```python
from build123d import *

# Parameters (mm, degrees)
MODEL_R             = 14.351
MODEL_R_2           = 2.413
MODEL_R_3           = 14.2875
BOSS_EXTRUDE1_DEPTH = 7.874
CUT_EXTRUDE3_REACH  = 9.874
SKETCH29_R          = 2.032
SKETCH29_R_2        = 9.525
CUT_EXTRUDE4_REACH  = 9.874
SKETCH34_R          = 2.4892
CUT_EXTRUDE5_REACH  = 9.874
SKETCH40_R          = 2.4892


with BuildPart() as part:
    # Model → Boss-Extrude1 (new body)
    with BuildSketch(Plane.XY):
        with BuildLine():
            Line((-44.522451968, 230.070582963), (-200.005250584, 313.419470721))
            ThreePointArc((-200.005250584, 313.419470721), (-219.438743814, 318.210854709), (-236.308771814, 307.439588539))
            Line((-236.308771814, 307.439588539), (-425.925316767, 28.829603592))
            ThreePointArc((-425.925316767, 28.829603592), (-430.312243104, 13.671313347), (-424.900993017, -1.152223962))
            Line((-424.900993017, -1.152223962), (-385.581467186, -51.204797614))
            ThreePointArc((-385.581467186, -51.204797614), (-376.711879358, -58.358090396), (-365.607528193, -60.913979882))
            Line((-365.607528193, -60.913979882), (-324.737451002, -60.913979882))
            ThreePointArc((-324.737451002, -60.913979882), (-318.798508014, -59.439796386), (-314.23831963, -55.359484793))
            Line((-314.23831963, -55.359484793), (-212.899365952, 93.541257838))
            ThreePointArc((-212.899365952, 93.541257838), (-203.778989185, 101.701881024), (-191.901103209, 104.650248016))
            Line((-191.901103209, 104.650248016), (48.661197018, 104.650248016))
            ThreePointArc((48.661197018, 104.650248016), (64.032332507, 99.471232012), (73.135172194, 86.046168785))
            Line((73.135172194, 86.046168785), (86.727013732, 37.098218434))
            ThreePointArc((86.727013732, 37.098218434), (106.362581421, 15.501750179), (127.326236921, 35.811553418))
            Line((127.326236921, 35.811553418), (140.807890588, 110.809453484))
            ThreePointArc((140.807890588, 110.809453484), (138.675228362, 126.361225539), (127.809114586, 137.689660276))
            Line((127.809114586, 137.689660276), (-44.522451968, 230.070582963))
        make_face()
        with Locations((-323.775189267, -35.513979882)):
            Circle(MODEL_R, mode=Mode.SUBTRACT)
        with Locations((-399.975189267, 2.586020118)):
            Circle(MODEL_R, mode=Mode.SUBTRACT)
        with Locations((107.006236921, 23.111553418)):
            Circle(MODEL_R_2, mode=Mode.SUBTRACT)
        with Locations((94.306236921, 35.811553418)):
            Circle(MODEL_R_2, mode=Mode.SUBTRACT)
        Polygon((110.67241113, 42.161553418), (114.33858534, 35.811553418), (110.67241113, 29.461553418), (103.340062712, 29.461553418), (99.673888502, 35.811553418), (103.340062712, 42.161553418), (107.006236921, 42.161553418), align=None, mode=Mode.SUBTRACT)
        with Locations((119.706236921, 35.811553418)):
            Circle(MODEL_R_2, mode=Mode.SUBTRACT)
        with Locations((107.006236921, 48.511553418)):
            Circle(MODEL_R_2, mode=Mode.SUBTRACT)
        with Locations((-190.707148919, 138.516914683)):
            Circle(MODEL_R, mode=Mode.SUBTRACT)
        with Locations((-208.832932893, 283.437784316)):
            Circle(MODEL_R, mode=Mode.SUBTRACT)
        with Locations((-40.935516122, 193.433854171)):
            Circle(MODEL_R_3, mode=Mode.SUBTRACT)
    extrude(amount=BOSS_EXTRUDE1_DEPTH)

    # Sketch29 → Cut-Extrude3 (cut, up to next)
    with BuildSketch(Plane.XY.offset(7.874), mode=Mode.PRIVATE) as cut_extrude3_sk1:
        with Locations((-182.711721066, 249.056735353)):
            Circle(SKETCH29_R)
    cut_extrude3_tool1 = extrude(cut_extrude3_sk1.sketch, amount=-CUT_EXTRUDE3_REACH, mode=Mode.PRIVATE) & part.part
    add(cut_extrude3_tool1.solids().sort_by_distance((-182.711721, 249.056735, 7.874))[0], mode=Mode.SUBTRACT)
    # Sketch29 → Cut-Extrude3 (cut, up to next)
    with BuildSketch(Plane.XY.offset(7.874), mode=Mode.PRIVATE) as cut_extrude3_sk2:
        with Locations((-134.081376724, 263.744472048)):
            Circle(SKETCH29_R)
    cut_extrude3_tool2 = extrude(cut_extrude3_sk2.sketch, amount=-CUT_EXTRUDE3_REACH, mode=Mode.PRIVATE) & part.part
    add(cut_extrude3_tool2.solids().sort_by_distance((-134.081377, 263.744472, 7.874))[0], mode=Mode.SUBTRACT)
    # Sketch29 → Cut-Extrude3 (cut, up to next)
    with BuildSketch(Plane.XY.offset(7.874), mode=Mode.PRIVATE) as cut_extrude3_sk3:
        with Locations((-165.740417242, 280.715775871)):
            Circle(SKETCH29_R)
    cut_extrude3_tool3 = extrude(cut_extrude3_sk3.sketch, amount=-CUT_EXTRUDE3_REACH, mode=Mode.PRIVATE) & part.part
    add(cut_extrude3_tool3.solids().sort_by_distance((-165.740417, 280.715776, 7.874))[0], mode=Mode.SUBTRACT)
    # Sketch29 → Cut-Extrude3 (cut, up to next)
    with BuildSketch(Plane.XY.offset(7.874), mode=Mode.PRIVATE) as cut_extrude3_sk4:
        with Locations((-151.052680548, 232.08543153)):
            Circle(SKETCH29_R)
    cut_extrude3_tool4 = extrude(cut_extrude3_sk4.sketch, amount=-CUT_EXTRUDE3_REACH, mode=Mode.PRIVATE) & part.part
    add(cut_extrude3_tool4.solids().sort_by_distance((-151.052681, 232.085432, 7.874))[0], mode=Mode.SUBTRACT)
    # Sketch29 → Cut-Extrude3 (cut, up to next)
    with BuildSketch(Plane.XY.offset(7.874), mode=Mode.PRIVATE) as cut_extrude3_sk5:
        with Locations((-158.396548895, 256.400603701)):
            Circle(SKETCH29_R_2)
    cut_extrude3_tool5 = extrude(cut_extrude3_sk5.sketch, amount=-CUT_EXTRUDE3_REACH, mode=Mode.PRIVATE) & part.part
    add(cut_extrude3_tool5.solids().sort_by_distance((-158.396549, 256.400604, 7.874))[0], mode=Mode.SUBTRACT)

    # Sketch34 → Cut-Extrude4 (cut, up to next)
    with BuildSketch(Plane.XY.offset(7.874), mode=Mode.PRIVATE) as cut_extrude4_sk1:
        with Locations((-228.733222311, 245.210842485)):
            Circle(SKETCH34_R)
    cut_extrude4_tool1 = extrude(cut_extrude4_sk1.sketch, amount=-CUT_EXTRUDE4_REACH, mode=Mode.PRIVATE) & part.part
    add(cut_extrude4_tool1.solids().sort_by_distance((-228.733222, 245.210842, 7.874))[0], mode=Mode.SUBTRACT)
    # Sketch34 → Cut-Extrude4 (cut, up to next)
    with BuildSketch(Plane.XY.offset(7.874), mode=Mode.PRIVATE) as cut_extrude4_sk2:
        with Locations((-249.731485055, 259.501852308)):
            Circle(SKETCH34_R)
    cut_extrude4_tool2 = extrude(cut_extrude4_sk2.sketch, amount=-CUT_EXTRUDE4_REACH, mode=Mode.PRIVATE) & part.part
    add(cut_extrude4_tool2.solids().sort_by_distance((-249.731485, 259.501852, 7.874))[0], mode=Mode.SUBTRACT)
    # Sketch34 → Cut-Extrude4 (cut, up to next)
    with BuildSketch(Plane.XY.offset(7.874), mode=Mode.PRIVATE) as cut_extrude4_sk3:
        with Locations((-391.784122689, 50.779120634)):
            Circle(SKETCH34_R)
    cut_extrude4_tool3 = extrude(cut_extrude4_sk3.sketch, amount=-CUT_EXTRUDE4_REACH, mode=Mode.PRIVATE) & part.part
    add(cut_extrude4_tool3.solids().sort_by_distance((-391.784123, 50.779121, 7.874))[0], mode=Mode.SUBTRACT)
    # Sketch34 → Cut-Extrude4 (cut, up to next)
    with BuildSketch(Plane.XY.offset(7.874), mode=Mode.PRIVATE) as cut_extrude4_sk4:
        with Locations((-370.785859945, 36.488110812)):
            Circle(SKETCH34_R)
    cut_extrude4_tool4 = extrude(cut_extrude4_sk4.sketch, amount=-CUT_EXTRUDE4_REACH, mode=Mode.PRIVATE) & part.part
    add(cut_extrude4_tool4.solids().sort_by_distance((-370.78586, 36.488111, 7.874))[0], mode=Mode.SUBTRACT)

    # Sketch40 → Cut-Extrude5 (cut, up to next)
    with BuildSketch(Plane(origin=(0, 0, 0), x_dir=(-1, 0, 0), z_dir=(0, 0, -1)), mode=Mode.PRIVATE) as cut_extrude5_sk1:
        with Locations((88.612396107, 240.73693678)):
            Circle(SKETCH40_R)
    cut_extrude5_tool1 = extrude(cut_extrude5_sk1.sketch, amount=-CUT_EXTRUDE5_REACH, mode=Mode.PRIVATE) & part.part
    add(cut_extrude5_tool1.solids().sort_by_distance((-88.612396, 240.736937, 0))[0], mode=Mode.SUBTRACT)
    # Sketch40 → Cut-Extrude5 (cut, up to next)
    with BuildSketch(Plane(origin=(0, 0, 0), x_dir=(-1, 0, 0), z_dir=(0, 0, -1)), mode=Mode.PRIVATE) as cut_extrude5_sk2:
        with Locations((154.68970629, 117.473322969)):
            Circle(SKETCH40_R)
    cut_extrude5_tool2 = extrude(cut_extrude5_sk2.sketch, amount=-CUT_EXTRUDE5_REACH, mode=Mode.PRIVATE) & part.part
    add(cut_extrude5_tool2.solids().sort_by_distance((-154.689706, 117.473323, 0))[0], mode=Mode.SUBTRACT)
    # Sketch40 → Cut-Extrude5 (cut, up to next)
    with BuildSketch(Plane(origin=(0, 0, 0), x_dir=(-1, 0, 0), z_dir=(0, 0, -1)), mode=Mode.PRIVATE) as cut_extrude5_sk3:
        with Locations((240.850237606, 132.8680637)):
            Circle(SKETCH40_R)
    cut_extrude5_tool3 = extrude(cut_extrude5_sk3.sketch, amount=-CUT_EXTRUDE5_REACH, mode=Mode.PRIVATE) & part.part
    add(cut_extrude5_tool3.solids().sort_by_distance((-240.850238, 132.868064, 0))[0], mode=Mode.SUBTRACT)
    # Sketch40 → Cut-Extrude5 (cut, up to next)
    with BuildSketch(Plane(origin=(0, 0, 0), x_dir=(-1, 0, 0), z_dir=(0, 0, -1)), mode=Mode.PRIVATE) as cut_extrude5_sk4:
        with Locations((261.829815531, 225.169665851)):
            Circle(SKETCH40_R)
    cut_extrude5_tool4 = extrude(cut_extrude5_sk4.sketch, amount=-CUT_EXTRUDE5_REACH, mode=Mode.PRIVATE) & part.part
    add(cut_extrude5_tool4.solids().sort_by_distance((-261.829816, 225.169666, 0))[0], mode=Mode.SUBTRACT)


solid = part.part
```
Build history of the part. All positions in model axes, mm. A direction names the side the tool comes from. Give positions to 0.01 mm unless a question says otherwise; leave off trailing zeros. Loops run counter-clockwise (first coordinate to the right, second up) from the corner with the lowest first, then second, coordinate; pieces in that order, holes last. Notation, with made-up numbers: (20, 59.25) -> (75, 59.25) arc R31 ccw to (75, 98.25) -> close; hole circle Ø2 at (40.5, 2.25). An arc over 180 degrees is marked (long way). One line per question, with ' | ' between items. Start each with the question number.
1) Two-plate mould, pull along X, no slides. Class faces 3 (the cylindrical face through (-219.154, 318.256, 3.882)), 4 (the cylindrical face through (138.77, 126.16, 3.88)), 5 (the cylindrical face through (105.91, 15.52, 3.88)): released by +X, released by -X, zero draft, split by the parting line, or undercut.
2) Probe L1, parallel to X at y = 119, z = 4.75; L2, parallel to Y at x = -315.5, z = 1.5; L3, parallel to Y at x = -206, z = 0.5. List the from-to ranges inside material, lowest first.
3) Pin check, flat tips, straight feed: pin 1 (7.5 mm diameter, centred on x = 107.01, y = 48.51, fed in from -Z); pin 2 (2.5 mm diameter, centred on x = -39, z = 3.5, fed in from -Y); pin 3 (1 mm diameter, centred on x = -222.5, z = 2, fed in from +Y); pin 4 (4 mm diameter, centred on y = 95, z = 4, fed in from -X). Stop position of each tip, or through.
4) Cut at B-B (x = 17.5). Give the cut face in (y, z), plus the area to 3 significant figures.
5) Cut at A-A (z = 1.25). Count the separate pieces of the cut face and the enclosed holes in it, plus the area to 3 significant figures.
6) 3-axis set-ups, long thin cutter, end or side, ignore diameter. For faces 1 (the flat face through (-149, 131, 0)), 2 (the cylindrical face through (63.85, 99.61, 3.88)): which of +Z, -Z, +X, -X, +Y, -Y reach the whole face in a straight line?
7) Cut at C-C (x = -70.5). Give the cut face in (y, z).
Return value:
1) face 3: split by the parting line | face 4: released by +X | face 5: undercut
2) L1: -364.56 to -156.66, -152.72 to 140.94 | L2: -56.93 to -47.24, -23.79 to 191.08 | L3: 100.38 to 269.37, 297.51 to 316.78
3) pin 1: z = 0 | pin 2: y = 104.65 | pin 3: y = 317.65 | pin 4: x = -382.25
4) outline: (104.65, 0) -> (196.82, 0) -> (196.82, 7.87) -> (104.65, 7.87) -> close | area: 726 mm^2
5) separate pieces: 1 | enclosed holes: 23 | area: 86,100 mm^2
6) face 1: -Z, +X, -X, +Y, -Y | face 2: +Z, -Z, -Y
7) outline: (104.65, 0) -> (244, 0) -> (244, 7.87) -> (104.65, 7.87) -> close
